Model file for the job. Use its own axes, mm. Face numbers are marked on the shaded views. A direction names the side the tool comes from. Coordinates: 2 decimals unless noted, no trailing zeros. Loops run counter-clockwise (first coordinate to the right, second up) from the corner with the lowest first, then second, coordinate; pieces in that order, holes last. Notation, with made-up numbers: M 37.5,82 L 61.5,82 A30 cw 61.5,115 Z; hole C 84.5,80 d9. An arc over 180 degrees is marked long. One line per question, with ' | ' between items. Start each with the question number.
```python
from build123d import *

# Parameters (mm, degrees)
EXTRUDE_1_DEPTH     = 5
SKETCH_2_R          = 1.5
CUT_EXTRUDE_1_DEPTH = 47.049538543
SKETCH_3_R          = 3
CUT_EXTRUDE_2_DEPTH = 3
FILLET_1_R          = 10
FILLET_2_R          = 1
CHAMFER_1_SIZE      = 1.5
SKETCH_4_W          = 3
SKETCH_4_H          = 10
SKETCH_4_W_2        = 3.010676302
CUT_EXTRUDE_3_DEPTH = 0.5


with BuildPart() as part:
    # 草图1 → 凸台-拉伸1 (new, symmetric)
    with BuildSketch(Plane.XY):
        Polygon((0, 0), (-14.549226784, 8.4), (-45, 8.4), (-45, 0), align=None)
    extrude(amount=EXTRUDE_1_DEPTH, both=True)

    # 草图2 → 切除-拉伸1 (cut, through all)
    with BuildSketch(Plane(origin=(0, 8.4, 0), x_dir=(1, 0, 0), z_dir=(0, 1, 0))):
        with Locations(Location((-39, 0, 0), (0, 0, 180))):
            Circle(SKETCH_2_R)
        with Locations(Location((-19, 0, 0), (0, 0, 180))):
            Circle(SKETCH_2_R)
    extrude(amount=-CUT_EXTRUDE_1_DEPTH, mode=Mode.SUBTRACT)

    # 草图3 → 切除-拉伸2 (cut)
    with BuildSketch(Plane(origin=(0, 8.4, 0), x_dir=(1, 0, 0), z_dir=(0, 1, 0))):
        with Locations(Location((-39, 0, 0), (0, 0, 180))):
            Circle(SKETCH_3_R)
        with Locations(Location((-19, 0, 0), (0, 0, 180))):
            Circle(SKETCH_3_R)
    extrude(amount=-CUT_EXTRUDE_2_DEPTH, mode=Mode.SUBTRACT)

    # 圆角1
    # the kernel refuses this fillet: 10 mm, written as the material it takes off along each edge
    with BuildSketch(Plane(origin=(-14.549226784, 8.4, -11.698729811), x_dir=(0.8660254037844417, -0.4999999999999948, 0), z_dir=(0, 0, 1))) as fillet_1_piece_1:
        with BuildLine():
            CenterArc((FILLET_1_R * 0.267949192431, -FILLET_1_R), FILLET_1_R, 90, 30)
            Line((-FILLET_1_R * 0.232050807569, -FILLET_1_R * 0.133974596216), (0, 0))
            Line((0, 0), (FILLET_1_R * 0.267949192431, 0))
        make_face()
    extrude(amount=23.397459622, mode=Mode.SUBTRACT)

    # 圆角2
    fillet_2_edges = [part.edges().sort_by_distance(p)[0] for p in [
        (0, 0, 0),
    ]]
    fillet(fillet_2_edges, radius=FILLET_2_R)

    # 倒角1
    chamfer_1_edges = [part.edges().sort_by_distance(p)[0] for p in [
        (-45, 0, 0),
        (-45, 8.4, 0),
    ]]
    chamfer(chamfer_1_edges, length=CHAMFER_1_SIZE)

    # 草图4 → 切除-拉伸3 (cut)
    with BuildSketch(Plane.XZ):
        with Locations((-39, 0)):
            Rectangle(SKETCH_4_W, SKETCH_4_H)
        with Locations((-19, 0)):
            Rectangle(SKETCH_4_W_2, SKETCH_4_H)
    extrude(amount=-CUT_EXTRUDE_3_DEPTH, mode=Mode.SUBTRACT)


solid = part.part
```
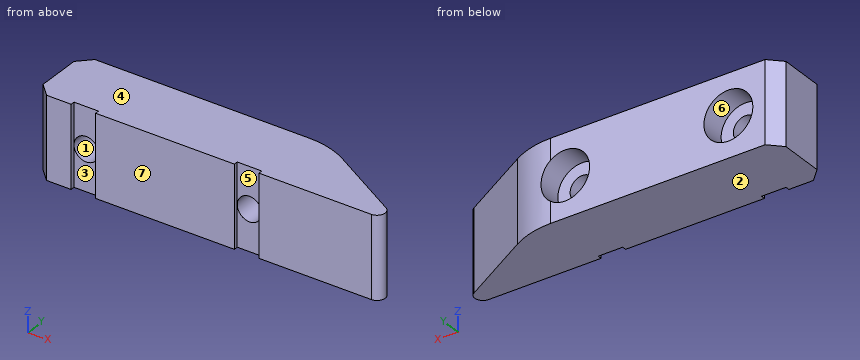
(1) Band-saw the part on A-A on x = -39. Write the cut outline in (y, z), then the cut area to 3 significant figures.
(2) Pin check, flat tips, straight feed: P1, Ø5.5, axis at x = -39, z = 0, coming from the +Y side; P2, Ø1.5, axis at x = -38.5, z = -1.5, coming from the -Y side; P3, Ø5, axis at x = -14, z = -2, coming from the +Y side. Stop position of each tip, or through.
(3) 3-axis set-ups, long thin cutter, end or side, ignore diameter. For the marked faces 5, 6 and 7: which of +Z, -Z, +X, -X, +Y, -Y reach the whole face in a straight line?
(4) Band-saw the part on C-C on y = 1. Write the cut outline in (x, z).
(5) Band-saw the part on B-B on z = -0.5. Give the number of separate pieces and of enclosed holes in the cut face, then the cut area to 3 significant figures.
(6) Two-plate mould, pull along Z, no slides. Class the marked faces 1, 2, 3 and 4: pulls with the +Z half, pulls with the -Z half, needs draft (parallel to the pull), parting line crosses it, or undercut.
(7) Band-saw the part on D-D on x = -19.5. Write the cut outline in (y, z), then the cut area to 3 significant figures.
(8) Drill centre lines: line 1 (Z direction, x = -19, y = 1.8); line 2 (X direction, y = 5, z = -0.25); line 3 (X direction, y = 2, z = 1). Where is each one in solid material? Low to high. Write a range as [from, to].
Computed values:
1) outline: M 0.5,-5 L 8.4,-5 L 8.4,-3 L 5.4,-3 L 5.4,-1.5 L 0.5,-1.5 Z; M 0.5,1.5 L 5.4,1.5 L 5.4,3 L 8.4,3 L 8.4,5 L 0.5,5 Z | area: 46.3 mm^2
2) P1: y = 5.4 | P2: y = 0.5 | P3: y = 8.37
3) face 5: +Z, -Z, -Y | face 6: +Y | face 7: +Z, -Z, +X, -X, -Y
4) outline: M -44.5,-5 L -2.73,-5 L -2.73,5 L -44.5,5 Z; hole C -39,0 d3; hole C -19,0 d3
5) separate pieces: 3 | enclosed holes: 0 | area: 245 mm^2
6) face 1: undercut | face 2: pulls with the -Z half | face 3: needs draft | face 4: pulls with the +Z half
7) outline: M 0.5,-5 L 8.4,-5 L 8.4,-2.96 L 5.4,-2.96 L 5.4,-1.41 L 0.5,-1.41 Z; M 0.5,1.41 L 5.4,1.41 L 5.4,2.96 L 8.4,2.96 L 8.4,5 L 0.5,5 Z | area: 47.4 mm^2
8) line 1: [-5, -1.5], [1.5, 5] | line 2: [-45, -40.48], [-37.52, -20.48], [-17.52, -8.66] | line 3: [-45, -40.12], [-37.88, -20.12], [-17.88, -3.46]
